The model under review builds one solid part; all positions refer to its coordinate system, in mm. A direction names the side the tool comes from. Coordinates: 2 decimals unless noted, no trailing zeros. Write each loop counter-clockwise with the first axis right and the second up, starting at its lowest first coordinate (ties: lowest second). Pieces come first, ordered by that corner, then holes. Notation, with made-up numbers: (21, 66.5) - (66, 66.5) arc R17 ccw to (66, 72.5) - close; hole circle Ø7 at (49.25, 1). An arc over 180 degrees is marked (long way). Answer as CSV lines item,"result". Start each with the question number.
```python
from build123d import *

# Parameters (mm, degrees)
SKETCH_1_R          = 2
EXTRUDE_1_DEPTH     = 36
SKETCH_2_R          = 6.5
EXTRUDE_2_DEPTH     = 5
SKETCH_3_R          = 6.5
EXTRUDE_3_DEPTH     = 15
EXTRUDE_3_TAPER     = 6
CUT_EXTRUDE_START   = -13
SKETCH_4_R          = 2
CUT_EXTRUDE_1_DEPTH = 13
FILLET_1_R          = 0.6


with BuildPart() as part:
    # 草图1 → 凸台-拉伸1 (new body)
    with BuildSketch(Plane.XY):
        Circle(SKETCH_1_R)
    extrude(amount=EXTRUDE_1_DEPTH)

    # 草图2 → 凸台-拉伸2 (add)
    with BuildSketch(Plane.XY.offset(16)):
        Circle(SKETCH_2_R)
    extrude(amount=EXTRUDE_2_DEPTH)

    # 草图3 → 凸台-拉伸3 (add)
    with BuildSketch(Plane.XY.offset(21)):
        Circle(SKETCH_3_R)
    extrude(amount=EXTRUDE_3_DEPTH, taper=EXTRUDE_3_TAPER)

    # 草图4 → 切除-拉伸1 (cut)
    with BuildSketch(Plane.XY.offset(36).offset(CUT_EXTRUDE_START)):
        Circle(SKETCH_4_R)
    extrude(amount=CUT_EXTRUDE_1_DEPTH, mode=Mode.SUBTRACT)

    # 圆角1
    fillet_1_edges = [part.edges().sort_by_distance(p)[0] for p in [
        (-4.923436471, 0, 36),
    ]]
    fillet(fillet_1_edges, radius=FILLET_1_R)


solid = part.part
```
(1) For pin 1 (3 mm diameter, centred on y = -3, z = 30.5, fed in from -X); pin 2 (1.5 mm diameter, centred on x = -1, y = 5, fed in from -Z); pin 3 (1 mm diameter, centred on x = 5, y = -1.5, fed in from +Z), all flat-tipped, find the tip position at first contact; note any pin that passes through.
(2) Add section C-C on z = 15. Give the boundary of the cut face in (x, y).
(3) Wall thickness on line 1 (Z direction, x = -0.25, y = 3); line 2 (Y direction, x = 0, z = 27); line 3 (Y direction, x = 0, z = 25.75): over which ranges is each line inside the solid? List them lowest first.
(4) For faces 4 (the flat face through (0, 0, 0)), 5 (the cylindrical face through (0, -2, 29)), list the 3-axis set-ups (+Z, -Z, +X, -X, +Y, -Y) from which the entire face can be reached by the end or side of a thin tool; tool diameter is ignored.
(5) The part is to be moulded in two halves that separate along X. For faces 1 (the flat face through (0, 0, 23)), 2 (the flat face through (1, 2, 16)), 3 (the cylindrical face through (0, -2, 8)), say which applies: released by +X, released by -X, zero draft, split by the parting line, or undercut.
(6) Add section A-A on x = 0. Give the boundary of the cut face in (y, z).
Reported:
1,pin 1,"x = -5.32"
1,pin 2,"z = 16"
1,pin 3,"z = 35.9"
2,outline,"circle Ø4 at (0, 0)"
3,line 1,"16 to 36"
3,line 2,"-5.87 to -2, 2 to 5.87"
3,line 3,"-6 to -2, 2 to 6"
4,face 4,"-Z, +X, -X, +Y, -Y"
4,face 5,"+Z"
5,face 1,"undercut"
5,face 2,"zero draft"
5,face 3,"split by the parting line"
6,outline,"(-6.5, 16) - (-2, 16) - (-2, 0) - (2, 0) - (2, 16) - (6.5, 16) - (6.5, 21) - (4.98, 35.46) arc R0.6 ccw to (4.38, 36) - (2, 36) - (2, 23) - (-2, 23) - (-2, 36) - (-4.38, 36) arc R0.6 ccw to (-4.98, 35.46) - (-6.5, 21) - close"
